from build123d import *

# Parameters (mm, degrees)
BOSS_EXTRUDE1_DEPTH = 50
SKETCH2_R           = 5
SKETCH2_W           = 245
SKETCH2_H           = 30
CUT_EXTRUDE1_DEPTH  = 351.356960827
FILLET1_R           = 15


with BuildPart() as part:
    # Sketch1 → Boss-Extrude1 (new body)
    with BuildSketch(Plane.XY):
        Polygon((-345, 25), (-255, 25), (-255, 10), (-345, 10), (-345, 0), (0, 0), (0, 35), (-345, 35), align=None)
    extrude(amount=BOSS_EXTRUDE1_DEPTH)

    # Sketch2 → Cut-Extrude1 (cut, through all)
    with BuildSketch(Plane(origin=(0, 35, 0), x_dir=(1, 0, 0), z_dir=(0, 1, 0))):
        with Locations(Location((-325, -25, 0), (0, 0, 180))):
            Circle(SKETCH2_R)
        with Locations((-132.5, -25)):
            Rectangle(SKETCH2_W, SKETCH2_H)
    extrude(amount=-CUT_EXTRUDE1_DEPTH, mode=Mode.SUBTRACT)

    # Fillet1
    fillet1_edges = [part.edges().sort_by_distance(p)[0] for p in [
        (-345, 30, 0),
        (-345, 30, 50),
        (-345, 5, 50),
        (-345, 5, 0),
    ]]
    fillet(fillet1_edges, radius=FILLET1_R)


solid = part.part
Here's how the part is built. I have some questions about the finished solid (model axes, mm). A direction names the side the tool comes from. Coordinates: 2 decimals unless noted, no trailing zeros. Order: outer loops, then holes, each group sorted by start corner. A loop starts at its lowest first (then second) coordinate and runs counter-clockwise, first axis right, second up. Notation, with made-up numbers: M 48.5,1.25 L 55.5,1.25 A34 cw 55.5,36.25 Z; hole C 19.5,66 d2. An arc over 180 degrees is marked long. Answer as CSV lines item,"result".
Item 1: Imagine slicing it at A-A on z = 25. Write out the boundary of the cut face in (x, y).
Results found:
outline,"M -345,0 L -330,0 L -330,10 L -345,10 Z; M -345,25 L -330,25 L -330,35 L -345,35 Z; M -320,0 L -255,0 L -255,10 L -320,10 Z; M -320,25 L -255,25 L -255,35 L -320,35 Z; M -10,0 L 0,0 L 0,35 L -10,35 Z"
Item 2: Imagine slicing it at D-D on x = -82. Write out the boundary of the cut face in (y, z), plus the area to 3 significant figures.
Results found:
outline,"M 0,0 L 35,0 L 35,10 L 0,10 Z; M 0,40 L 35,40 L 35,50 L 0,50 Z"
area,"700 mm2"
Item 3: Imagine slicing it at B-B on x = -325. Write out the boundary of the cut face in (y, z), plus the area to 3 significant figures.
Results found:
outline,"M 0,0 L 10,0 L 10,20 L 0,20 Z; M 0,30 L 10,30 L 10,50 L 0,50 Z; M 25,0 L 35,0 L 35,20 L 25,20 Z; M 25,30 L 35,30 L 35,50 L 25,50 Z"
area,"800 mm2"
Item 4: If I drill on line 1 (Z direction, x = -325, y = 7.5); line 2 (Z direction, x = -88.5, y = 12.5); line 3 (Y direction, x = -315, z = 21), over which ranges is the centre line in solid material (lowest first)?
Results found:
line 1,"0 to 20, 30 to 50"
line 2,"0 to 10, 40 to 50"
line 3,"0 to 10, 25 to 35"
Item 5: We'd pull the mould along Y, two halves only. Please class faces 4 (the face through (-301, 25, 25)), 5 (the face through (-340.72, 29.93, 45.49)), 6 (the face through (-208, 35, 41)): +Y half, -Y half, draft (parallel to the pull), parting line (faces both ways), or undercut.
Results found:
face 4,"undercut"
face 5,"draft"
face 6,"+Y half"
Item 6: For pin 1 (8 mm diameter, centred on y = 17.5, z = 46, fed in from -X); pin 2 (1.5 mm diameter, centred on y = 28.5, z = 7, fed in from -X), each with a flat end and sliding along its axis, tell me the tip position at first contact or that it passes through.
Results found:
pin 1,"x = -255"
pin 2,"x = -343.13"
Item 7: Imagine slicing it at C-C on y = 6. Write out the boundary of the cut face in (x, z).
Results found:
outline,"M -345,15 A15 ccw -330,0 L 0,0 L 0,50 L -330,50 A15 ccw -345,35 Z; hole C -325,25 d10; hole M -255,10 L -10,10 L -10,40 L -255,40 Z"
Item 8: On a 3-axis mill with a long thin cutter (end or side, diameter ignored), from which of +Z, -Z, +X, -X, +Y, -Y can I reach the whole of each face in a straight line? I mean faces 1 (the face through (-255, 18, 5)), 2 (the face through (-134, 18, 10)), 3 (the face through (-340.72, 29.93, 4.51)). Say none if no direction works.
Results found:
face 1,"+Z, -Z, -X"
face 2,"+Y, -Y"
face 3,"-Z, -X, +Y, -Y"
